Design review of the part built by this model. Coordinates are the model's own, in mm. A direction names the side the tool comes from. Round coordinates to 2 decimals unless told otherwise and drop trailing zeros. Write each loop counter-clockwise with the first axis right and the second up, starting at its lowest first coordinate (ties: lowest second). Pieces come first, ordered by that corner, then holes.
Autodesk Inventor part; units mm, degrees
ref_plane "Work Plane1" through (0, 33, 0) normal (0, 1, 0) x (1, 0, 0)
ref_plane "YZ Plane" through (0, 0, 0) normal (1, 0, 0) x (0, 1, 0)
ref_plane "XZ Plane" through (0, 0, 0) normal (0, 1, 0) x (-1, 0, 0)
sketch "Sketch1" plane through (0, 0, 0) normal (0, 1, 0) x (-1, 0, 0)
  circle A0 centre (0, 0) radius 60
  dimension "d0" = 120
extrude "Extrusion1" add sketch "Sketch1" along normal blind 3
ref_plane "Work Plane1" through (0, 33, 0) normal (0, 1, 0) x (1, 0, 0)
sketch "Sketch2" plane through (0, 33, 0) normal (0, 1, 0) x (1, 0, 0)
  circle A0 centre (0, 0) radius 5
  dimension "d5" = 10
loft "Loft1" add profiles "Sketch2" section 1 edges at (60, 3, 0)
sketch "Sketch3" plane through (0, 0, 0) normal (0, -1, 0) x (1, 0, 0)
  circle A0 centre (0, 0) radius 6.5
  dimension "d10" = 13
extrude "Extrusion2" cut sketch "Sketch3" against normal blind 16
sketch "Sketch5" plane through (0, 33, 0) normal (0, 1, 0) x (1, 0, 0)
  circle A0 centre (0, 0) radius 2.75
  dimension "d16" = 5.5
extrude "Extrusion4" cut sketch "Sketch5" against normal through all
sketch "Sketch6" plane through (0, 33, 0) normal (0, 1, 0) x (1, 0, 0)
  line L0 (0, 4.6188) -> (4, 2.3094)
  line L1 (4, 2.3094) -> (4, -2.3094)
  line L2 (4, -2.3094) -> (0, -4.6188)
  line L3 (0, -4.6188) -> (-4, -2.3094)
  line L4 (-4, -2.3094) -> (-4, 2.3094)
  line L5 (-4, 2.3094) -> (0, 4.6188)
  point P0 (0, 0)
  point P1 (0, 0)
  dimension "d19" = 8
extrude "Extrusion5" cut sketch "Sketch6" against normal blind 4
properties part number "Bottom_Foot"
1) Add section B-B on y = 4.5. State the section outline as (x, z) points.
2) For P1, Ø1.5, axis at y = 16.5, z = 11, coming from the +X side; P2, Ø6, axis at y = 23.5, z = 13.5, coming from the +X side; P3, Ø1.5, axis at x = 7, y = 8.5, coming from the -Z side; P4, Ø3.5, axis at x = 0, z = 0, coming from the +Y side, all flat-tipped, find the tip position at first contact; note any pin that passes through.
3) The part is to be moulded in two halves that separate along X. For faces 1 (the face through (59.94, 1.48, -2.64)), 2 (the face through (1.97, 31.03, -3.48)), 3 (the face through (-3, 29, 1)), 4 (the face through (1, 0, -12)), say which applies: pulls with the +X half, pulls with the -X half, needs draft (parallel to the pull), parting line crosses it, or undercut.
4) For faces 5 (the face through (3, 16, 0)), 6 (the face through (-2.028, 31.028, -3.448)), 7 (the face through (2, 33, -4)), list the 3-axis set-ups (+Z, -Z, +X, -X, +Y, -Y) from which the entire face can be reached by the end or side of a thin tool; tool diameter is ignored.
5) For line 1 along Z through (x, y) = (0, 8.25) (3 decimals); line 2 along Z through (x, y) = (0, 4.25); line 3 along X through (y, z) = (22, 0), list the stretches that pass through material, from the lowest coordinate up.
6) Add section A-A on y = 22.5. State the section outline as (x, z) points, and give its area (3 significant figures).
Computed:
1. outline: circle Ø114.5 at (0, 0); hole circle Ø13 at (0, 0)
2. P1: stops at x = 34.95
2. P2: stops at x = 24.64
2. P3: stops at z = -50.82
2. P4: passes through
3. face 1: parting line crosses it
3. face 2: undercut
3. face 3: undercut
3. face 4: needs draft
4. face 5: -Y
4. face 6: +Y
4. face 7: +Z, -Z, +X, -X, +Y
5. line 1: z = -50.375 to -6.5, 6.5 to 50.375
5. line 2: z = -57.71 to -6.5, 6.5 to 57.71
5. line 3: x = -25.17 to -2.75, 2.75 to 25.17
6. outline: circle Ø48.5 at (0, 0); hole circle Ø5.5 at (0, 0)
6. area: 1,820 mm2
